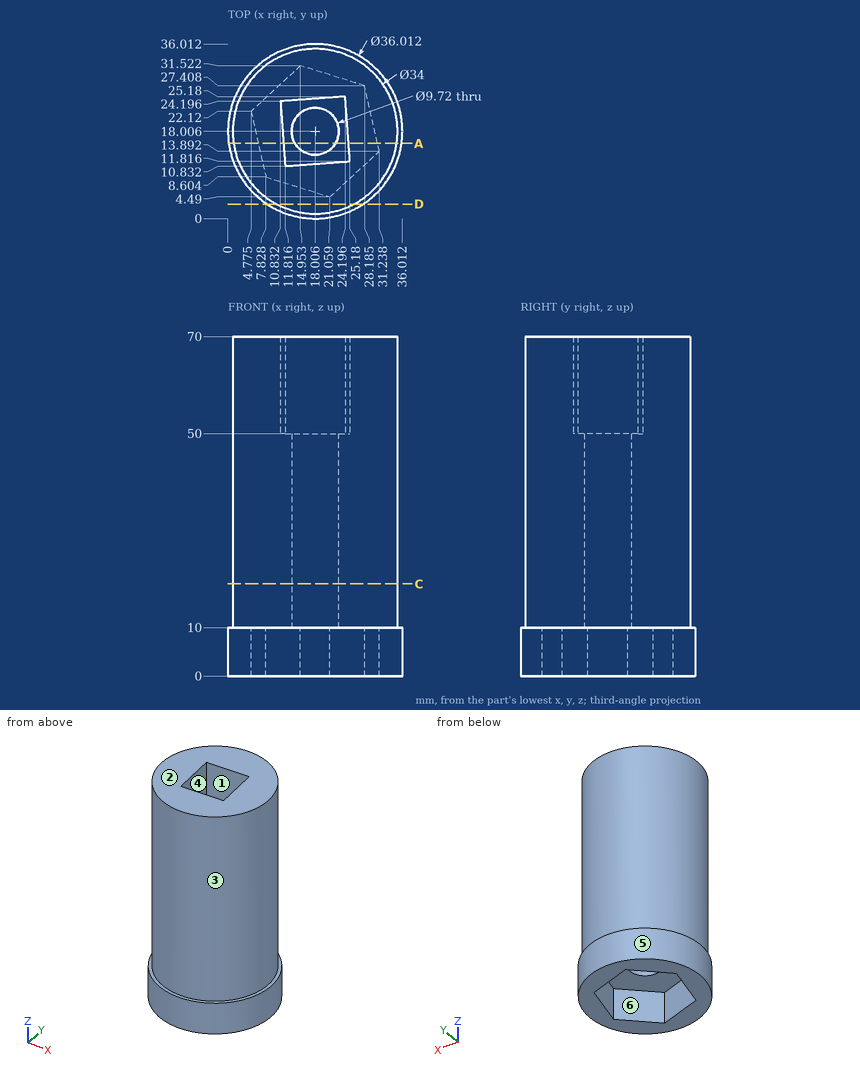
Verification items for this drawing (mm, ordinates from the low corner). A direction names the side the tool comes from. Coordinates: 2 decimals unless noted, no trailing zeros. Loops run counter-clockwise (first coordinate to the right, second up) from the corner with the lowest first, then second, coordinate; pieces in that order, holes last. Notation, with made-up numbers: (87, 17) - (117, 17) arc R33 ccw to (117, 47) - close; hole circle Ø11 at (60, -23.5). An arc over 180 degrees is marked (long way). Use one line per item in the form item = value. Start each with the question number.
Item 1: Thickness scan on probe 1 along X at (y, z) = (19.5, 55.5) (1 decimal); probe 2 along Z at (x, y) = (13.5, 10); probe 3 along X at (y, z) = (16.5, 36) (1 decimal). Record the ranges inside material, lowest first.
Item 2: Section check A-A, the plane y = 15.5. Enter the section's corners in (x, z) (1 decimal), and give its area (3 significant figures).
Item 3: Gauge pin test, flat ends, axial feed: pin 1 (1 mm diameter, centred on x = 11, y = 18, fed in from -Z); pin 2 (8 mm diameter, centred on x = 27.5, z = 23, fed in from -Y); pin 3 (5 mm diameter, centred on x = 18, z = 55, fed in from -Y). Record the tip position at first contact, or that the pin passes through.
Item 4: Section check D-D, the plane y = 3. Enter the section's corners in (x, z) (1 decimal).
Item 5: Section check C-C, the plane z = 19. Enter the section's corners in (x, y).
Item 6: Tool access check on the marked faces 4, 5 and 6. Record the directions out of +Z, -Z, +X, -X, +Y, -Y that give a thin tool (end or side, any length) a straight path to the whole face; none if there is none.
Item 7: Mould release check, pull along X, two halves, no side actions. Record for the marked faces 1, 2 and 3: +X half, -X half, draft (parallel to the pull), parting line (faces both ways), or undercut.
Computed:
q1.probe_1 = 1.1 to 11.2, 24.6 to 34.9
q1.probe_2 = 10 to 70
q1.probe_3 = 1.1 to 13.4, 22.6 to 34.9
q2.outline = (0.2, 0) - (6.3, 0) - (6.3, 10) - (13.8, 10) - (13.8, 50) - (11.5, 50) - (11.5, 70) - (1.2, 70) - (1.2, 10) - (0.2, 10) - close; (22.2, 10) - (30.9, 10) - (30.9, 0) - (35.8, 0) - (35.8, 10) - (34.8, 10) - (34.8, 70) - (24.9, 70) - (24.9, 50) - (22.2, 50) - close
q2.area = 1,530 mm2
q3.pin_1 = 10
q3.pin_2 = 1.92
q3.pin_3 = 1.01
q4.outline = (8.1, 0) - (28, 0) - (28, 10) - (26, 10) - (26, 70) - (10, 70) - (10, 10) - (8.1, 10) - close
q5.outline = circle Ø34 at (18.01, 18.01); hole circle Ø9.72 at (18.01, 18.01)
q6.face_4 = +Z
q6.face_5 = +Z, -Z
q6.face_6 = -Z
q7.face_1 = undercut
q7.face_2 = draft
q7.face_3 = parting line
